Read the model definition and answer for the solid it produces. Units are mm, in the model's axes. A direction names the side the tool comes from. Coordinates: 2 decimals unless noted, no trailing zeros. Write each loop counter-clockwise with the first axis right and the second up, starting at its lowest first coordinate (ties: lowest second). Pieces come first, ordered by that corner, then holes. Notation, with made-up numbers: (17.5, -37.5) -> (41.5, -37.5) arc R27 ccw to (41.5, -21.5) -> close; hole circle Ø3 at (76, -37). An arc over 180 degrees is marked (long way). Use CSV: the item, a comma, the result in double quotes. Start each with the question number.
from build123d import *

# Parameters (mm, degrees)
SKETCH_5_R          = 5
SKETCH_5_R_2        = 1.5
EXTRUDE_1_DEPTH     = 20
SKETCH_6_R          = 2.15
CUT_EXTRUDE_3_DEPTH = 20
CUT_EXTRUDE_START   = -20
SKETCH_7_R          = 2.15
CUT_EXTRUDE_4_DEPTH = 20
SKETCH_8_W          = 33.77726644
SKETCH_8_H          = 35
CUT_EXTRUDE_5_DEPTH = 10
SKETCH_9_R          = 9.75
CUT_EXTRUDE_6_DEPTH = 6.2
CHAMFER_1_SIZE      = 3
SKETCH_12_W         = 110.408141216
SKETCH_12_H         = 73.303439967
CUT_EXTRUDE_8_DEPTH = 20
SKETCH_13_W         = 20.5
SKETCH_13_H         = 20
EXTRUDE_2_DEPTH     = 0.25
SKETCH_14_W         = 20
SKETCH_14_H         = 40.25
SKETCH_14_R         = 2.15
EXTRUDE_3_DEPTH     = 0.25


with BuildPart() as part:
    # 草图5 → 凸台-拉伸1 (new body)
    with BuildSketch(Plane.XY):
        Polygon((0, 0), (0, 50), (72, 50), (72, 15), (30.5, 15), (30.5, 0), (25.5, 0), (25.5, 40.5), (5, 40.5), (5, 0), align=None)
        with Locations((55.25, 32.5)):
            Circle(SKETCH_5_R, mode=Mode.SUBTRACT)
        with Locations((43.25, 44.5)):
            Circle(SKETCH_5_R_2, mode=Mode.SUBTRACT)
        with Locations((67.25, 44.5)):
            Circle(SKETCH_5_R_2, mode=Mode.SUBTRACT)
        with Locations((43.25, 20.5)):
            Circle(SKETCH_5_R_2, mode=Mode.SUBTRACT)
        with Locations((67.25, 20.5)):
            Circle(SKETCH_5_R_2, mode=Mode.SUBTRACT)
    extrude(amount=EXTRUDE_1_DEPTH)

    # 草图6 → 切除-拉伸3 (cut)
    with BuildSketch(Plane.ZY):
        with Locations((10, 10.25)):
            Circle(SKETCH_6_R)
        with Locations((10, 30.25)):
            Circle(SKETCH_6_R)
    extrude(amount=-CUT_EXTRUDE_3_DEPTH, mode=Mode.SUBTRACT)

    # 草图7 → 切除-拉伸4 (cut)
    with BuildSketch(Plane(origin=(30.5, 0, 0), x_dir=(0, 0, -1), z_dir=(1, 0, 0)).offset(CUT_EXTRUDE_START)):
        with Locations(Location((-10, 10.25, 0), (0, 0, 180))):
            Circle(SKETCH_7_R)
    extrude(amount=CUT_EXTRUDE_4_DEPTH, mode=Mode.SUBTRACT)

    # 草图8 → 切除-拉伸5 (cut)
    with BuildSketch(Plane(origin=(0, 0, 0), x_dir=(-1, 0, 0), z_dir=(0, 0, -1))):
        with Locations((-55.11136678, 32.5)):
            Rectangle(SKETCH_8_W, SKETCH_8_H)
    extrude(amount=-CUT_EXTRUDE_5_DEPTH, mode=Mode.SUBTRACT)

    # 草图9 → 切除-拉伸6 (cut)
    with BuildSketch(Plane(origin=(0, 0, 10), x_dir=(-1, 0, 0), z_dir=(0, 0, -1))):
        with Locations((-55.25, 32.5)):
            Circle(SKETCH_9_R)
    extrude(amount=-CUT_EXTRUDE_6_DEPTH, mode=Mode.SUBTRACT)

    # 倒角1
    chamfer_1_edges = [part.edges().sort_by_distance(p)[0] for p in [
        (0, 50, 10),
        (72, 50, 15),
        (72, 15, 15),
        (38.22273356, 32.5, 0),
    ]]
    chamfer(chamfer_1_edges, length=CHAMFER_1_SIZE)


with BuildPart() as body_2:
    # 镜向1: mirrored copy
    add(part.part.mirror(Plane(origin=(0, 0, 20), x_dir=(1, 0, 0), z_dir=(0, 0, -1))))

    # 草图13 → 凸台-拉伸2 (add)
    with BuildSketch(Plane.XZ.offset(-40.5)):
        with Locations((15.25, 30)):
            Rectangle(SKETCH_13_W, SKETCH_13_H)
    extrude(amount=EXTRUDE_2_DEPTH)

    # 草图14 → 凸台-拉伸3 (add)
    with BuildSketch(Plane(origin=(5, 0, 0), x_dir=(0, 0, -1), z_dir=(1, 0, 0))):
        with Locations((-30, 20.125)):
            Rectangle(SKETCH_14_W, SKETCH_14_H)
        with Locations((-30, 10.25)):
            Circle(SKETCH_14_R, mode=Mode.SUBTRACT)
        with Locations((-30, 30.25)):
            Circle(SKETCH_14_R, mode=Mode.SUBTRACT)
    extrude(amount=EXTRUDE_3_DEPTH)


with BuildPart() as part_1:
    add(part.part)

    # 草图12 → 切除-拉伸8 (cut)
    with BuildSketch(Plane(origin=(0, 0, 0), x_dir=(-1, 0, 0), z_dir=(0, 0, -1))):
        with Locations((-31.097159048, 24.893638624)):
            Rectangle(SKETCH_12_W, SKETCH_12_H)
    extrude(amount=-CUT_EXTRUDE_8_DEPTH, mode=Mode.SUBTRACT)


solid = body_2.part
1) Each of these flat-tipped pins is pushed along its axis until it touches: pin 1 (4 mm diameter, centred on y = 10.25, z = 30, fed in from -X); pin 2 (10 mm diameter, centred on x = 50.5, y = 31, fed in from +Z); pin 3 (1 mm diameter, centred on y = 16.5, z = 28, fed in from +X); pin 4 (7.5 mm diameter, centred on y = 39.5, z = 35, fed in from +X). Where does it stop, or does it pass through?
2) Find the intervals of material crossed by line 1 along X through (y, z) = (44.5, 28); line 2 along Y through (x, z) = (43.25, 25); line 3 along X through (y, z) = (27.5, 33.5), in increasing order.
3) Section C-C, the plane y = 44.5 is taken. Give the vertices of the cut face in (x, z).
4) Section D-D, the plane x = 43.25 is taken. Give the vertices of the cut face in (y, z).
5) Section B-B, the plane z = 22.5 is taken. Give the vertices of the cut face in (x, y), plus the area to 3 significant figures.
6) The mould has two halves that part along Y. Classify faces 6 (the face through (28, 50, 28)), 7 (the face through (71, 17, 25)), 8 (the face through (62.99, 26.57, 26.94)), 9 (the face through (36.74, 32.26, 38.48)): pulls with the +Y half, pulls with the -Y half, needs draft (parallel to the pull), parting line crosses it, or undercut.
7) Section A-A, the plane y = 10.25 is taken. Give the vertices of the cut face in (x, z), plus the area to 3 significant figures.
8) Which of the six approach directions +Z, -Z, +X, -X, +Y, -Y give full straight-line access (tool end or side, diameter ignored) to faces 1 (the face through (25.5, 20, 30)), 2 (the face through (48, 41, 30)), 3 (the face through (50.255, 32.72, 21.927)), 4 (the face through (2.59, 32.06, 28.84)), 5 (the face through (2, 49, 30))?
The answers:
1,pin 1,"passes through"
1,pin 2,"stops at z = 30"
1,pin 3,"stops at x = 71"
1,pin 4,"stops at x = 38.22"
2,line 1,"x = 0 to 41.75, 44.75 to 65.75, 68.75 to 72"
2,line 2,"y = 15 to 19, 22 to 43, 46 to 50"
2,line 3,"x = 0 to 5.25, 25.5 to 38.22"
3,outline,"(0, 20) -> (41.75, 20) -> (41.75, 30) -> (38.22, 30) -> (38.22, 37) -> (35.22, 40) -> (0, 40) -> close; (44.75, 20) -> (65.75, 20) -> (65.75, 30) -> (44.75, 30) -> close; (68.75, 20) -> (72, 20) -> (72, 30) -> (68.75, 30) -> close"
4,outline,"(15, 20) -> (19, 20) -> (19, 30) -> (15, 30) -> close; (22, 20) -> (43, 20) -> (43, 30) -> (22, 30) -> close; (46, 20) -> (50, 20) -> (50, 30) -> (46, 30) -> close"
5,outline,"(0, 0) -> (5.25, 0) -> (5.25, 40.25) -> (25.5, 40.25) -> (25.5, 0) -> (30.5, 0) -> (30.5, 15) -> (69, 15) -> (72, 18) -> (72, 47) -> (69, 50) -> (3, 50) -> (0, 47) -> close; hole circle Ø3 at (43.25, 20.5); hole circle Ø3 at (43.25, 44.5); hole circle Ø10 at (55.25, 32.5); hole circle Ø3 at (67.25, 20.5); hole circle Ø3 at (67.25, 44.5)"
5,area,"2,040 mm^2"
6,face 6,"pulls with the +Y half"
6,face 7,"pulls with the -Y half"
6,face 8,"undercut"
6,face 9,"needs draft"
7,outline,"(0, 20) -> (5.25, 20) -> (5.25, 27.85) -> (0, 27.85) -> close; (0, 32.15) -> (5.25, 32.15) -> (5.25, 40) -> (0, 40) -> close; (25.5, 20) -> (30.5, 20) -> (30.5, 27.85) -> (25.5, 27.85) -> close; (25.5, 32.15) -> (30.5, 32.15) -> (30.5, 40) -> (25.5, 40) -> close"
7,area,"161 mm^2"
8,face 1,"+Z, -Z, -Y"
8,face 2,"+Z, +X, +Y, -Y"
8,face 3,"+Z, -Z"
8,face 4,"-X"
8,face 5,"+Z, -Z, -X, +Y"
